from build123d import *

# Parameters (mm, degrees)
SKETCH1_R           = 3
BOSS_EXTRUDE1_DEPTH = 2.5


with BuildPart() as part:
    # Sketch1 → Boss-Extrude1 (new body, symmetric)
    with BuildSketch(Plane.XY):
        with BuildLine():
            Line((-90, 5.5), (90, 5.5))
            ThreePointArc((90, 5.5), (95.5, 0), (90, -5.5))
            Line((90, -5.5), (-90, -5.5))
            ThreePointArc((-90, -5.5), (-95.5, 0), (-90, 5.5))
        make_face()
        with Locations((-90, 0)):
            Circle(SKETCH1_R, mode=Mode.SUBTRACT)
        with Locations((90, 0)):
            Circle(SKETCH1_R, mode=Mode.SUBTRACT)
        with Locations((50, 0)):
            Circle(SKETCH1_R, mode=Mode.SUBTRACT)
    extrude(amount=BOSS_EXTRUDE1_DEPTH, both=True)


solid = part.part
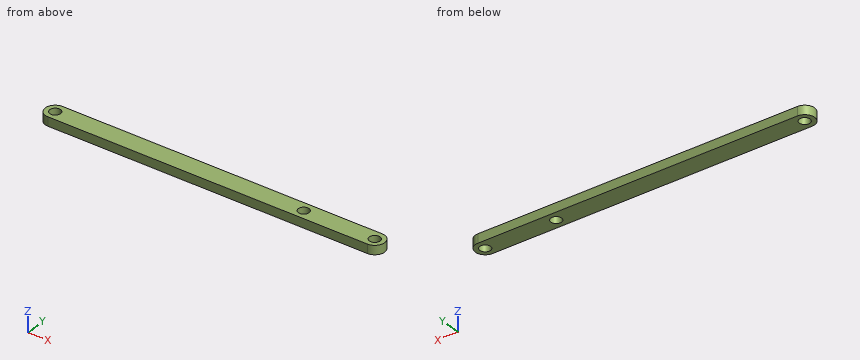
Geometry check sheet. Reference: the model listing, model coordinates, mm. Give positions to 0.01 mm unless a question says otherwise; leave off trailing zeros. Loops run counter-clockwise (first coordinate to the right, second up) from the corner with the lowest first, then second, coordinate; pieces in that order, holes last.
(1) Thickness scan on L1, parallel to Y at x = -90, z = -0.4; L2, parallel to X at y = 0.5, z = -2.2; L3, parallel to X at y = 0.75, z = -1. Record the ranges inside material, lowest first.
From the geometry:
L1: y = -5.5 to -3, 3 to 5.5
L2: x = -95.48 to -92.96, -87.04 to 47.04, 52.96 to 87.04, 92.96 to 95.48
L3: x = -95.45 to -92.9, -87.1 to 47.1, 52.9 to 87.1, 92.9 to 95.45
(2) Section check A-A on x = 50. Record the cut outline in (y, z).
From the geometry:
outline: (-5.5, -2.5) - (-3, -2.5) - (-3, 2.5) - (-5.5, 2.5) - close; (3, -2.5) - (5.5, -2.5) - (5.5, 2.5) - (3, 2.5) - close
(3) Depth check by flat-ended pin: pin 1 Ø1 at (y, z) = (-3, -1) entering from +X. Enter the tip coordinate at first touch or a pass-through.
From the geometry:
pin 1: stops at x = 94.9
(4) Section check B-B on z = 0.5. Record the cut outline in (x, y), then the cut area to 3 significant figures.
From the geometry:
outline: (-90, -5.5) - (90, -5.5) arc R5.5 ccw to (90, 5.5) - (-90, 5.5) arc R5.5 ccw to start; hole circle Ø6 at (-90, 0); hole circle Ø6 at (50, 0); hole circle Ø6 at (90, 0)
area: 1,990 mm2
